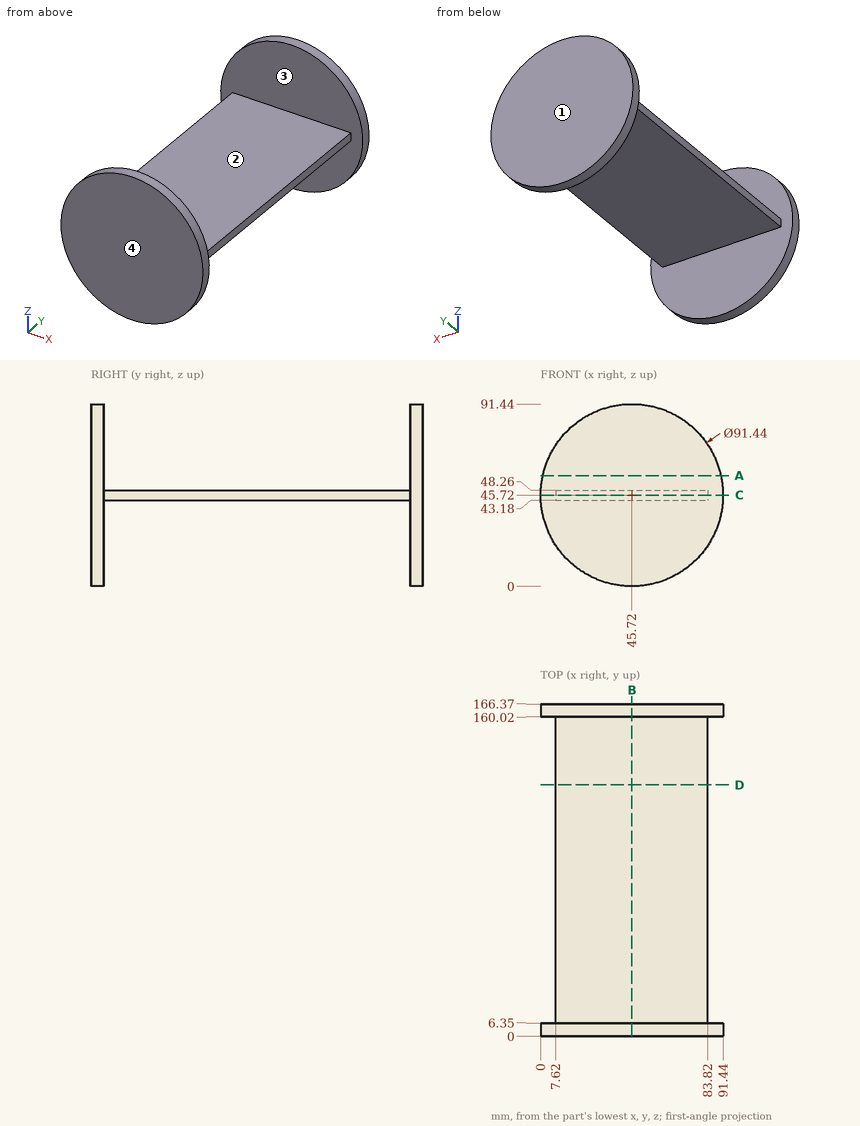
The drawing under review shows one solid part. Ordinate dimensions are in mm from its lowest x, y, z. Coordinates: 2 decimals unless noted, no trailing zeros. Order: outer loops, then holes, each group sorted by start corner. A loop starts at its lowest first (then second) coordinate and runs counter-clockwise, first axis right, second up. Notation, with made-up numbers: (75, 2.25) -> (83, 2.25) arc R30 cw to (83, 31.25) -> close; hole circle Ø7 at (-25.5, -3.75). An arc over 180 degrees is marked (long way). Return JSON: item names as keys, results as strings.
1. We need section B-B on x = 45.72. Write out the cut boundary in (y, z), and give its area (3 significant figures).
Answer block:
{"outline": "(0, 0) -> (6.35, 0) -> (6.35, 43.18) -> (160.02, 43.18) -> (160.02, 0) -> (166.37, 0) -> (166.37, 91.44) -> (160.02, 91.44) -> (160.02, 48.26) -> (6.35, 48.26) -> (6.35, 91.44) -> (0, 91.44) -> close", "area": "1,940 mm²"}
2. The part is to be moulded in two halves that separate along Y. For the marked faces 1, 2, 3 and 4, say which applies: +Y half, -Y half, draft (parallel to the pull), parting line (faces both ways), or undercut.
Answer block:
{"face 1": "+Y half", "face 2": "undercut", "face 3": "undercut", "face 4": "-Y half"}
3. For pin 1 Ø23 at (x, y) = (48.5, 101) entering from +Z; pin 2 Ø10 at (x, y) = (44, 148.5) entering from -Z; pin 3 Ø1.5 at (y, z) = (103.5, 46) entering from -X; pin 4 Ø12 at (x, z) = (72, 62.5) entering from -Y, all flat-tipped, find the tip position at first contact; note any pin that passes through.
Answer block:
{"pin 1": "z = 48.26", "pin 2": "z = 43.18", "pin 3": "x = 7.62", "pin 4": "y = 0"}
4. We need section D-D on y = 126. Write out the cut boundary in (x, z).
Answer block:
{"outline": "(7.62, 43.18) -> (83.82, 43.18) -> (83.82, 48.26) -> (7.62, 48.26) -> close"}
5. We need section C-C on z = 45.72. Write out the cut boundary in (x, y).
Answer block:
{"outline": "(0, 0) -> (91.44, 0) -> (91.44, 6.35) -> (83.82, 6.35) -> (83.82, 160.02) -> (91.44, 160.02) -> (91.44, 166.37) -> (0, 166.37) -> (0, 160.02) -> (7.62, 160.02) -> (7.62, 6.35) -> (0, 6.35) -> close"}
6. We need section A-A on z = 55.5. Write out the cut boundary in (x, y), and give its area (3 significant figures).
Answer block:
{"outline": "(1.06, 0) -> (90.38, 0) -> (90.38, 6.35) -> (1.06, 6.35) -> close; (1.06, 160.02) -> (90.38, 160.02) -> (90.38, 166.37) -> (1.06, 166.37) -> close", "area": "1,130 mm²"}
7. For line 1 (Y direction, x = 13, z = 49); line 2 (Z direction, x = 60, y = 27), list the stretches that pass through material, from the lowest coordinate up. Write a range as from..to.
Answer block:
{"line 1": "0..6.35, 160.02..166.37", "line 2": "43.18..48.26"}
